```python
from build123d import *

# Parameters (mm, degrees)
SKETCH1_W           = 86
SKETCH1_H           = 3
BOSS_EXTRUDE1_DEPTH = 10
SKETCH3_W           = 3
SKETCH3_H           = 3
CUT_EXTRUDE2_DEPTH  = 5
FILLET2_R           = 1


with BuildPart() as part:
    # Sketch1 → Boss-Extrude1 (new body)
    with BuildSketch(Plane.XY):
        with Locations((43, 1.5)):
            Rectangle(SKETCH1_W, SKETCH1_H)
    extrude(amount=BOSS_EXTRUDE1_DEPTH)

    # Sketch3 → Cut-Extrude2 (cut)
    with BuildSketch(Plane(origin=(0, 0, 0), x_dir=(-1, 0, 0), z_dir=(0, 0, -1))):
        with Locations((-79.5, 1.5)):
            Rectangle(SKETCH3_W, SKETCH3_H)
        with Locations((-58.5, 1.5)):
            Rectangle(SKETCH3_W, SKETCH3_H)
        with Locations((-38.5, 1.5)):
            Rectangle(SKETCH3_W, SKETCH3_H)
        with Locations((-22.5, 1.5)):
            Rectangle(SKETCH3_W, SKETCH3_H)
        with Locations((-4.7, 1.5)):
            Rectangle(SKETCH3_W, SKETCH3_H)
    extrude(amount=-CUT_EXTRUDE2_DEPTH, mode=Mode.SUBTRACT)

    # Fillet2
    fillet2_edges = [part.edges().sort_by_distance(p)[0] for p in [
        (78, 1.5, 0),
        (81, 1.5, 0),
        (57, 1.5, 0),
        (60, 1.5, 0),
        (37, 1.5, 0),
        (40, 1.5, 0),
        (21, 1.5, 0),
        (24, 1.5, 0),
        (3.2, 1.5, 0),
        (6.2, 1.5, 0),
    ]]
    fillet(fillet2_edges, radius=FILLET2_R)


solid = part.part
```
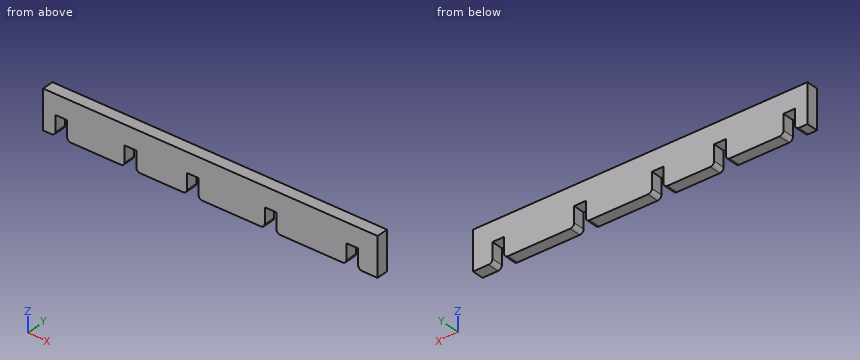
Geometry check sheet. Reference: the model listing, model coordinates, mm. Coordinates: 2 decimals unless noted, no trailing zeros. Loops run counter-clockwise (first coordinate to the right, second up) from the corner with the lowest first, then second, coordinate; pieces in that order, holes last.
Item 1: Thickness scan on line 1 (X direction, y = 1.95, z = 2); line 2 (Z direction, x = 38, y = 2.55); line 3 (Z direction, x = 3, y = 2.55). Record the ranges inside material, lowest first.
Item 2: Go/stop test with a flat-tipped pin: pin 1 Ø0.9 at (x, y) = (22.5, 1.5) entering from -Z. Record where the tip stops, or that it passes through.
Item 3: Sectioned sample at A-A, the plane z = 2. Record the boundary of the cut face in (x, y).
Check result:
1. line 1: x = 0 to 3.2, 6.2 to 21, 24 to 37, 40 to 57, 60 to 78, 81 to 86
1. line 2: z = 5 to 10
1. line 3: z = 0.4 to 10
2. pin 1: stops at z = 5
3. outline: (0, 0) - (3.2, 0) - (3.2, 3) - (0, 3) - close; (6.2, 0) - (21, 0) - (21, 3) - (6.2, 3) - close; (24, 0) - (37, 0) - (37, 3) - (24, 3) - close; (40, 0) - (57, 0) - (57, 3) - (40, 3) - close; (60, 0) - (78, 0) - (78, 3) - (60, 3) - close; (81, 0) - (86, 0) - (86, 3) - (81, 3) - close
